Check sheet for the modelled part. Datum: model origin and axes. Units: mm. Face numbers are marked on the shaded views. A direction names the side the tool comes from. Round coordinates to 2 decimals unless told otherwise and drop trailing zeros. Order: outer loops, then holes, each group sorted by start corner. A loop starts at its lowest first (then second) coordinate and runs counter-clockwise, first axis right, second up. Notation, with made-up numbers: (31.25, 46) -> (45.25, 46) arc R23 ccw to (45.25, 57) -> close; hole circle Ø10 at (17, -23). An arc over 180 degrees is marked (long way). Answer in a Markdown table with one row per item.
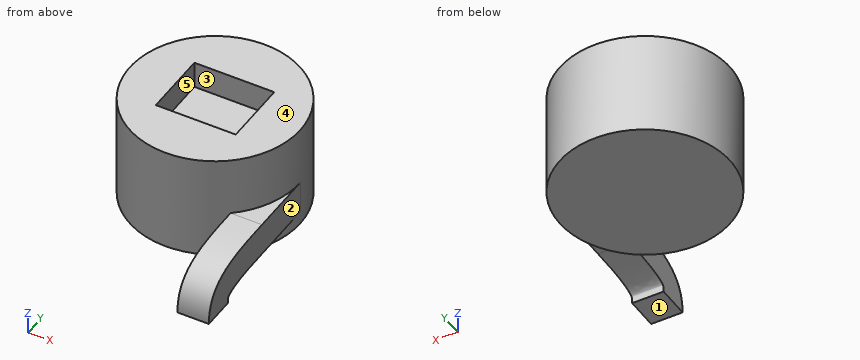
Autodesk Inventor part; units mm, degrees
ref_plane "Work Plane1" through (0, 0, 35) normal (0, 0, -1) x (-1, 0, 0)
ref_plane "Work Plane2" through (65, 0, 0) normal (1, 0, 0) x (0, 1, 0)
ref_plane "XZ Plane" through (0, 0, 0) normal (0, 1, 0) x (-1, 0, 0)
sketch "Sketch1" plane through (0, 0, 0) normal (0, 0, 1) x (1, 0, 0)
  circle A0 centre (0, 0) radius 65
  dimension "d0" = 130
extrude "Extrusion1" add sketch "Sketch1" along normal blind 80
ref_plane "Work Plane1" through (0, 0, 35) normal (0, 0, -1) x (-1, 0, 0)
ref_plane "Work Plane2" through (65, 0, 0) normal (1, 0, 0) x (0, 1, 0)
sketch "Sketch2" plane through (0, 0, 35) normal (0, 0, -1) x (-1, 0, 0)
  circle A0 centre (0, 0) radius 65
  line L0 (0, 0) -> (-65, 0) construction
  circle A1 centre (0, 0) radius 65
  line L1 (-65, 0) -> (-41, 0)
  line L2 (-41, 0) -> (-41, -50.4381)
  line L3 (-41, -50.4381) -> (-65, -50.4381)
  line L4 (-65, -50.4381) -> (-65, 0)
  dimension "d4" = 24
extrude "Extrusion2" add sketch "Sketch2" along normal blind 25 contours A0 L3 L4
sketch "Sketch3" plane through (65, 0, 0) normal (1, 0, 0) x (0, 1, 0)
  line L0 (0, 35) -> (-50.4381, 35)
  line L1 (-50.4381, 35) -> (-50.4381, 10)
  line L2 (0, 10) -> (-50.4381, 10) construction
  line L3 (0, 10) -> (0, 35) construction
  line L4 (0, 35) -> (-50.4381, 35)
  line L5 (-50.4381, 35) -> (-85.4381, 35) construction
  line L6 (-85.4381, 35) -> (-120.4381, 35) construction
  line L7 (-120.4381, 35) -> (-120.4381, 0) construction
  spline S0 degree 3 poles (-50.4381, 35) (-85.4381, 35) (-120.4381, 35) (-120.4381, 0) knots 1 1 1 1 2 2 2 2
  line L8 (0, 0) -> (-133.4667, 0) construction
  line L9 (-120.4381, 0) -> (-120.4381, 80.5106) construction
  line L10 (-50.4381, 35) -> (-166.769, 35) construction
  line L11 (111.3538, 35) -> (-213.1228, 35) construction
  dimension "d7" = 70
  dimension "d8" = 35
  dimension "d9" = 35
sketch "Sketch4" plane through (41, -50.4381, 35) normal (0, -1, 0) x (1, 0, 0)
  line L0 (24, 0) -> (0, 0)
  line L1 (0, -25) -> (0, 0)
  line L2 (24, -25) -> (0, -25)
  line L3 (24, 0) -> (24, -25)
  point P0 (-41, -35)
sweep "Sweep1" add profiles "Sketch4" path "Sketch3" path curves S0
sketch "Sketch5" plane through (0, 0, 80) normal (0, 0, 1) x (1, 0, 0)
  circle A0 centre (0, 0) radius 65
  line L0 (-30.48, 25.4) -> (30.48, 25.4)
  line L1 (30.48, 25.4) -> (30.48, -25.4)
  line L2 (30.48, -25.4) -> (-30.48, -25.4)
  line L3 (-30.48, -25.4) -> (-30.48, 25.4)
  line L4 (-30.48, 25.4) -> (30.48, -25.4) construction
  line L5 (30.48, 25.4) -> (-30.48, -25.4) construction
  dimension "d12" = 60.96
  dimension "d13" = 50.8
extrude "Extrusion3" cut sketch "Sketch5" against normal blind 20.663 contours L0 L1 L2 L3
properties part number "Dust Bin CFD"
Item 1: Cross-section at C-C (y = -41.5). Record the boundary of the cut face in (x, z).
Result sheet:
| item | result |
|---|---|
| outline | (-50.03, 0) -> (50.03, 0) -> (50.03, 10) -> (65, 10) -> (65, 35) -> (50.03, 35) -> (50.03, 80) -> (-50.03, 80) -> close |
Item 2: Depth check by flat-ended pin: P1, Ø8, axis at y = -10.5, z = 70, coming from the -X side; P2, Ø6, axis at y = 3, z = 65.5, coming from the +X side; P3, Ø10.5, axis at y = -5.5, z = 67.5, coming from the -X side; P4, Ø4, axis at x = 14.5, z = 41.5, coming from the +Y side. Enter the tip coordinate at first touch or a pass-through.
Result sheet:
| item | result |
|---|---|
| P1 | stops at x = -64.67 |
| P2 | stops at x = 65 |
| P3 | stops at x = -65 |
| P4 | stops at y = 63.79 |
Item 3: Cross-section at A-A (z = 65). Record the boundary of the cut face in (x, y).
Result sheet:
| item | result |
|---|---|
| outline | circle Ø130 at (0, 0); hole (-30.48, -25.4) -> (30.48, -25.4) -> (30.48, 25.4) -> (-30.48, 25.4) -> close |
Item 4: Mould release check, pull along X, two halves, no side actions. Record for the marked faces 1, 2 and 3: pulls with the +X half, pulls with the -X half, needs draft (parallel to the pull), parting line crosses it, or undercut.
Result sheet:
| item | result |
|---|---|
| face 1 | needs draft |
| face 2 | pulls with the +X half |
| face 3 | undercut |
Item 5: Cross-section at B-B (x = 0). Record the boundary of the cut face in (y, z), and give its area (3 significant figures).
Result sheet:
| item | result |
|---|---|
| outline | (-65, 0) -> (65, 0) -> (65, 80) -> (25.4, 80) -> (25.4, 59.34) -> (-25.4, 59.34) -> (-25.4, 80) -> (-65, 80) -> close |
| area | 9,350 mm^2 |
Item 6: Set-up check for the marked faces 4 and 5: record each of +Z, -Z, +X, -X, +Y, -Y from which the full face is reachable in a straight line by a thin tool's end or side.
Result sheet:
| item | result |
|---|---|
| face 4 | +Z, +X, -X, +Y, -Y |
| face 5 | +Z |
Item 7: Scan lines: line 1 (X direction, y = -102, z = 17); line 2 (X direction, y = 22, z = 70); line 3 (Y direction, x = 1, z = 15). Record each from-to range of solid material in increasing order. Write a range as [from, to].
Result sheet:
| item | result |
|---|---|
| line 1 | x = [41, 65] |
| line 2 | x = [-61.16, -30.48], [30.48, 61.16] |
| line 3 | y = [-64.99, 64.99] |
Item 8: Cross-section at D-D (z = 47). Record the boundary of the cut face in (x, y), and give its area (3 significant figures).
Result sheet:
| item | result |
|---|---|
| outline | circle Ø130 at (0, 0) |
| area | 13,300 mm^2 |
